Autodesk Inventor part; units mm, degrees
ref_plane "YZ Plane" through (0, 0, 0) normal (1, 0, 0) x (0, 1, 0)
ref_plane "XZ Plane" through (0, 0, 0) normal (0, 1, 0) x (-1, 0, 0)
ref_plane "XY Plane" through (0, 0, 0) normal (0, 0, 1) x (1, 0, 0)
sketch "Szkic1" plane through (0, 0, 0) normal (0, 0, 1) x (1, 0, 0)
  line L0 (0, 0) -> (0, 25)
  line L1 (0, 25) -> (6, 25)
  line L2 (6, 25) -> (6, 30.35)
  line L3 (6, 30.35) -> (23, 30.35)
  line L4 (23, 30.35) -> (23, 27.4)
  line L5 (23, 27.4) -> (39.5, 27.4)
  line L6 (39.5, 27.4) -> (39.5, 28.35)
  line L7 (39.5, 28.35) -> (46.7, 28.35)
  line L8 (46.7, 28.35) -> (46.7, 23)
  line L9 (46.7, 0) -> (0, 0)
  line L10 (46.7, 23) -> (41.45, 23)
  line L11 (41.45, 23) -> (41.45, 0)
  dimension "d0" = 25
  dimension "d1" = 6
  dimension "d3" = 30.35
  dimension "d4" = 17
  dimension "d5" = 27.4
  dimension "d6" = 16.5
  dimension "d7" = 7.2
  dimension "d8" = 28.35
  dimension "d10" = 5.25
  dimension "d11" = 23
revolve "Obrót1" add sketch "Szkic1" angle 360 about axis through (46.7, 0, 0) along (-1, 0, 0)
properties part number "obiektyw"
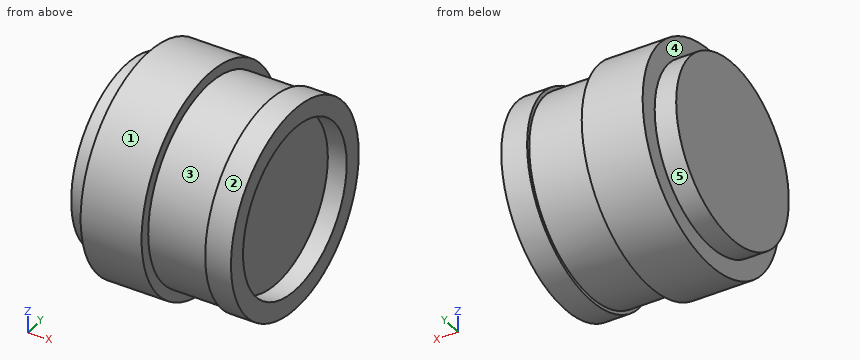
The listing builds one solid part. Answer for the finished solid, in the listing's coordinates (mm). Face numbers are marked on the shaded views. A direction names the side the tool comes from. Coordinates: 2 decimals unless noted, no trailing zeros. Order: outer loops, then holes, each group sorted by start corner. A loop starts at its lowest first (then second) coordinate and runs counter-clockwise, first axis right, second up.
Q1. A cutting plane is placed at C-C, the plane x = 8. Write down the section's boundary in (y, z).
Q2. Which of the six approach directions +Z, -Z, +X, -X, +Y, -Y give full straight-line access (tool end or side, diameter ignored) to the marked faces 1 and 2?
Q3. A cutting plane is placed at A-A, the plane z = 0. Write down the section's boundary in (x, y), and give its area (3 significant figures).
Q4. Consider line 1 (Z direction, x = 44, y = 0); line 2 (X direction, y = 7, z = -27). Determine where each line is inside the solid, lowest interval first.
Q5. For a pull along X with two mould halves and no side action, classify the marked faces 3, 4 and 5 as pulls with the +X half, pulls with the -X half, needs draft (parallel to the pull), parting line crosses it, or undercut.
Q6. Given P1, Ø12, axis at x = 22.5, y = -12, coming from the -Z side; P2, Ø4, axis at y = 17, z = 12, coming from the -X side; P3, Ø1.5, axis at x = 38, y = -11.5, coming from the +Z side; P4, Ø8, axis at x = 31, y = -2.5, coming from the -Z side, each flat-ended and moving along its own axis, determine where each tip first touches the part or whether it passes through.
Q7. A cutting plane is placed at D-D, the plane x = 24. Write down the section's boundary in (y, z).
Answers follow:
1. outline: circle Ø60.7 at (0, 0)
2. face 1: +X, -X
2. face 2: +X
3. outline: (0, -25) - (6, -25) - (6, -30.35) - (23, -30.35) - (23, -27.4) - (39.5, -27.4) - (39.5, -28.35) - (46.7, -28.35) - (46.7, -23) - (41.45, -23) - (41.45, 23) - (46.7, 23) - (46.7, 28.35) - (39.5, 28.35) - (39.5, 27.4) - (23, 27.4) - (23, 30.35) - (6, 30.35) - (6, 25) - (0, 25) - close
3. area: 2,400 mm2
4. line 1: z = -28.35 to -23, 23 to 28.35
4. line 2: x = 6 to 23, 39.5 to 46.7
5. face 3: undercut
5. face 4: pulls with the -X half
5. face 5: needs draft
6. P1: stops at z = -29.75
6. P2: stops at x = 0
6. P3: stops at z = 25.2
6. P4: stops at z = -27.4
7. outline: circle Ø54.8 at (0, 0)
